```python
from build123d import *

# Parameters (mm, degrees)
F0_W      = 45
F0_H      = 60
F1_DEPTH  = 5
F2_W      = 5
F2_H      = 60
F3_DEPTH  = 40
F4_SIZE2  = 20
F4_SIZE   = 20
F5_R      = 5
F6_DEPTH  = 50
F8_D      = 6
F8_DEPTH  = 20
F8_TIP    = 1.8025818571
F10_DEPTH = 2
F11_DEPTH = 2


# Not quite as in the source:
# - after a boolean that leaves OpenCascade's solid faulty, fix() repairs it


with BuildPart() as f1:
    # F0 (on Front) → F1 (new body)
    with BuildSketch(Plane.XZ):
        Rectangle(F0_W, F0_H)
    extrude(amount=F1_DEPTH)

    # F2 (on face) → F3 (join)
    with BuildSketch(Plane.XZ.offset(5)):
        with Locations((-20, 0)):
            Rectangle(F2_W, F2_H)
        with Locations((20, 0)):
            Rectangle(F2_W, F2_H)
    extrude(amount=F3_DEPTH)

    # F4
    f4_edges = [f1.edges().sort_by_distance(p)[0] for p in [
        (20, -45, 30),
        (-20, -45, 30),
        (20, -45, -30),
        (-20, -45, -30),
    ]]
    chamfer(f4_edges, length=F4_SIZE, length2=F4_SIZE2)

    # F5 (on face) → F6 (cut)
    with BuildSketch(Plane(origin=(-22.5, 0, 0), x_dir=(0, -1, 0), z_dir=(-1, 0, 0))):
        with Locations((30, 0)):
            Circle(F5_R)
    extrude(amount=-F6_DEPTH, mode=Mode.SUBTRACT)

    # F8
    with Locations(Plane.XZ.offset(5)):
        with Locations((0, 0)):
            Hole(F8_D / 2, depth=F8_DEPTH)
            with Locations((0, 0, -(F8_DEPTH + F8_TIP / 2))):  # 118° drill point
                Cone(0, F8_D / 2, F8_TIP, mode=Mode.SUBTRACT)

    # F9 (on face) → F10 (cut)
    with BuildSketch(Plane(origin=(0, 0, 0), x_dir=(-1, 0, 0), z_dir=(0, 1, 0))):
        with BuildLine():
            Line((-5, -1), (-3.7431358354, -1))
            ThreePointArc((-3.7431358354, -1), (-3.8701524892, 0), (-3.7431358354, 1))
            Line((-3.7431358354, 1), (-5, 1))
            Line((-5, 1), (-5, -1))
        make_face()
        with BuildLine():
            ThreePointArc((-1, 3.8371140982), (-0.0042634526, 3.997751149), (1, 3.9042073005))
            Line((1, 3.9042073005), (1, 5))
            Line((1, 5), (-1, 5))
            Line((-1, 5), (-1, 3.8371140982))
        make_face()
        with BuildLine():
            Line((4.002830857, -1), (5, -1))
            Line((5, -1), (5, 1))
            Line((5, 1), (4.002830857, 1))
            ThreePointArc((4.002830857, 1), (4.0979662959, 0.5040171699), (4.1298475108, 0))
            ThreePointArc((4.1298475108, 0), (4.0979662959, -0.5040171699), (4.002830857, -1))
        make_face()
        with BuildLine():
            Line((1, -5), (1, -3.9042073005))
            ThreePointArc((1, -3.9042073005), (-0.0042634526, -3.997751149), (-1, -3.8371140982))
            Line((-1, -3.8371140982), (-1, -5))
            Line((-1, -5), (1, -5))
        make_face()
    extrude(amount=-F10_DEPTH, mode=Mode.SUBTRACT)

    # F9 (on face) → F11 (cut)
    with BuildSketch(Plane(origin=(0, 0, 0), x_dir=(-1, 0, 0), z_dir=(0, 1, 0))):
        with BuildLine():
            Line((2.8284271247, -1), (4.002830857, -1))
            ThreePointArc((4.002830857, -1), (4.0979662959, -0.5040171699), (4.1298475108, 0))
            ThreePointArc((4.1298475108, 0), (4.0979662959, 0.5040171699), (4.002830857, 1))
            Line((4.002830857, 1), (2.8284271247, 1))
            ThreePointArc((2.8284271247, 1), (2.956795679, 0.5073059362), (3, 0))
            ThreePointArc((3, 0), (2.956795679, -0.5073059362), (2.8284271247, -1))
        make_face()
        with BuildLine():
            ThreePointArc((-3.7431358354, 1), (-3.8701524892, 0), (-3.7431358354, -1))
            Line((-3.7431358354, -1), (-2.8284271247, -1))
            ThreePointArc((-2.8284271247, -1), (-3, 0), (-2.8284271247, 1))
            Line((-2.8284271247, 1), (-3.7431358354, 1))
        make_face()
        with BuildLine():
            Line((1, 2.8284271247), (1, 3.9042073005))
            ThreePointArc((1, 3.9042073005), (-0.0042634526, 3.997751149), (-1, 3.8371140982))
            Line((-1, 3.8371140982), (-1, 2.8284271247))
            ThreePointArc((-1, 2.8284271247), (0, 3), (1, 2.8284271247))
        make_face()
        with BuildLine():
            ThreePointArc((-1, -3.8371140982), (-0.0042634526, -3.997751149), (1, -3.9042073005))
            Line((1, -3.9042073005), (1, -2.8284271247))
            ThreePointArc((1, -2.8284271247), (0, -3), (-1, -2.8284271247))
            Line((-1, -2.8284271247), (-1, -3.8371140982))
        make_face()
    extrude(amount=-F11_DEPTH, mode=Mode.SUBTRACT)

    add(f1.part.fix(), mode=Mode.REPLACE)


solid = f1.part
```
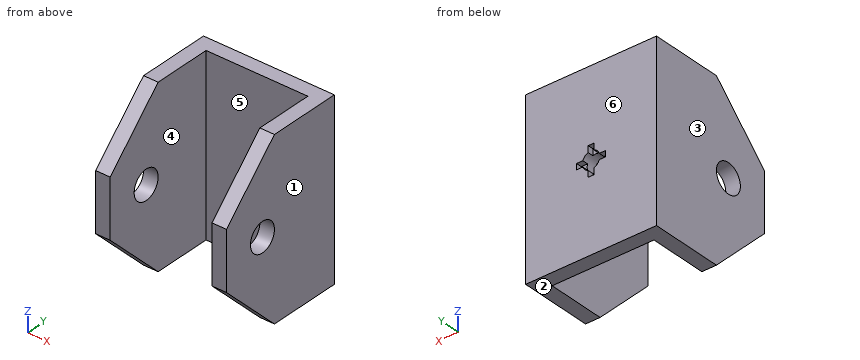
Here's how the part is built. I have some questions about the finished solid (model axes, mm). Face numbers are marked on the shaded views. A direction names the side the tool comes from. Coordinates: 2 decimals unless noted, no trailing zeros. Loops run counter-clockwise (first coordinate to the right, second up) from the corner with the lowest first, then second, coordinate; pieces in that order, holes last. Notation, with made-up numbers: (-37, 65) - (-31, 65) arc R19 cw to (-31, 97) - close; hole circle Ø3 at (54, 89.25). An arc over 180 degrees is marked (long way). Return JSON: item names as keys, results as strings. Group by question number.
Item 1: If we section it at C-C on x = 0: Write out the boundary of the cut face in (y, z), and give its area (3 significant figures).
Item 2: On a 3-axis mill with a long thin cutter (end or side, diameter ignored), from which of +Z, -Z, +X, -X, +Y, -Y can I reach the whole of each face in a straight line? I mean the marked faces 5 and 6. Say none if no direction works.
Item 3: If we section it at A-A on y = -23.5: Write out the boundary of the cut face in (x, z), and give its area (3 significant figures).
Item 4: I need wall thicknesses on line 1 (Z direction, x = 0, y = -1.8); line 2 (X direction, y = -24, z = 15.5); line 3 (X direction, y = -1.1, z = 0). Which ranges of each line are inside material? Lowest first, please. Write a range as from..to.
Item 5: We'd pull the mould along X, two halves only. Please class the marked faces 1, 2, 3 and 4: +X half, -X half, draft (parallel to the pull), parting line (faces both ways), or undercut.
Item 6: If we section it at B-B on z = 0: Write out the boundary of the cut face in (x, y).
Item 7: Will these pins go through, and if not, where does the flat tip stop? P1, Ø4, axis at x = -2, z = -4.5, coming from the -Y side; P2, Ø1.6, axis at x = 0.5, z = -3.5, coming from the +Y side.
Item 8: If we section it at D-D on y = -30: Write out the boundary of the cut face in (x, z).
Calculated:
{
 "1": {"outline": "(-5, -30) - (0, -30) - (0, -5) - (-2, -5) - (-2, -3) - (-5, -3) - close; (-5, 3) - (-2, 3) - (-2, 5) - (0, 5) - (0, 30) - (-5, 30) - close", "area": "262 mm^2"},
 "2": {"face 5": "+Z, -Z, -Y", "face 6": "+Z, -Z, +X, -X, +Y"},
 "3": {"outline": "(-22.5, -30) - (-17.5, -30) - (-17.5, 30) - (-22.5, 30) - close; (17.5, -30) - (22.5, -30) - (22.5, 30) - (17.5, 30) - close", "area": "600 mm^2"},
 "4": {"line 1": "z = -30..-5, 5..30", "line 2": "x = -22.5..-17.5, 17.5..22.5", "line 3": "x = -22.5..-5, 5..22.5"},
 "5": {"face 1": "+X half", "face 2": "draft", "face 3": "-X half", "face 4": "undercut"},
 "6": {"outline": "(-22.5, -45) - (-17.5, -45) - (-17.5, -35) - (-22.5, -35) - close; (-22.5, -25) - (-17.5, -25) - (-17.5, -5) - (-3, -5) - (-3, -2) - (-5, -2) - (-5, 0) - (-22.5, 0) - close; (3, -5) - (17.5, -5) - (17.5, -25) - (22.5, -25) - (22.5, 0) - (5, 0) - (5, -2) - (3, -2) - close; (17.5, -45) - (22.5, -45) - (22.5, -35) - (17.5, -35) - close"},
 "7": {"P1": "stops at y = -5", "P2": "stops at y = 0"},
 "8": {"outline": "(-22.5, -25) - (-17.5, -25) - (-17.5, -5) - (-22.5, -5) - close; (-22.5, 5) - (-17.5, 5) - (-17.5, 25) - (-22.5, 25) - close; (17.5, -25) - (22.5, -25) - (22.5, -5) - (17.5, -5) - close; (17.5, 5) - (22.5, 5) - (22.5, 25) - (17.5, 25) - close"}
}
